Design review of the part built by this model. Coordinates are the model's own, in mm. A direction names the side the tool comes from. Coordinates: 2 decimals unless noted, no trailing zeros. Write each loop counter-clockwise with the first axis right and the second up, starting at its lowest first coordinate (ties: lowest second). Pieces come first, ordered by that corner, then holes. Notation, with made-up numbers: (79.5, 86) - (86.5, 86) arc R22 cw to (86.5, 125) - close; hole circle Ø9 at (-31.75, 19). An arc over 180 degrees is marked (long way). Answer as a JSON object with one key per item and string values.
Autodesk Inventor part; units mm, degrees
ref_plane "YZ Plane" through (0, 0, 0) normal (1, 0, 0) x (0, 1, 0)
ref_plane "XZ Plane" through (0, 0, 0) normal (0, 1, 0) x (-1, 0, 0)
ref_plane "XY Plane" through (0, 0, 0) normal (0, 0, 1) x (1, 0, 0)
sketch "Boceto1" plane through (0, 0, 0) normal (0, 1, 0) x (-1, 0, 0)
  line L0 (0, 0) -> (250, 0)
  line L1 (250, 0) -> (250, -600)
  line L2 (250, -600) -> (0, -600)
  line L3 (0, -600) -> (0, 0)
  line L4 (250, 0) -> (250, -20)
  line L5 (250, -20) -> (0, -20)
  line L6 (0, 0) -> (20, 0)
  line L7 (20, 0) -> (20, -600)
  line L8 (0, -600) -> (0, -580)
  line L9 (0, -580) -> (250, -580)
  line L10 (250, -600) -> (230, -600)
  line L11 (230, -600) -> (230, 0)
  point P0 (20, -20)
  point P1 (20, -580)
  point P2 (230, -580)
  point P3 (230, -20)
  dimension "d0" = 250
  dimension "d1" = 600
  dimension "d2" = 20
  dimension "d3" = 20
  dimension "d4" = 20
  dimension "d5" = 20
extrude "Extrusión1" add sketch "Boceto1" along normal blind 1160 contours L0 L7 L5 L3 | L0 L1 L5 L11 | L9 L7 L2 L3 | L9 L1 L2 L11
extrude "Extrusión2" add sketch "Boceto1" along normal blind 1160 contours L0 L11 L5 L7 | L5 L7 L9 L3 | L5 L11 L9 L7 | L5 L1 L9 L11 | L9 L11 L2 L7
extrude "Extrusión3" cut sketch "Boceto1" along normal blind 1147.5 contours L0 L11 L5 L7 | L5 L7 L9 L3 | L5 L11 L9 L7 | L5 L1 L9 L11 | L9 L11 L2 L7
extrude "Extrusión4" add sketch "Boceto1" along normal blind 787.5 contours L0 L11 L5 L7 | L5 L7 L9 L3 | L5 L11 L9 L7 | L5 L1 L9 L11 | L9 L11 L2 L7
extrude "Extrusión5" cut sketch "Boceto1" along normal blind 775 contours L0 L11 L5 L7 | L5 L7 L9 L3 | L5 L11 L9 L7 | L5 L1 L9 L11 | L9 L11 L2 L7
extrude "Extrusión6" add sketch "Boceto1" along normal blind 470 contours L0 L11 L5 L7 | L5 L7 L9 L3 | L5 L11 L9 L7 | L5 L1 L9 L11 | L9 L11 L2 L7
extrude "Extrusión7" cut sketch "Boceto1" along normal blind 457.5 contours L0 L11 L5 L7 | L5 L7 L9 L3 | L5 L11 L9 L7 | L5 L1 L9 L11 | L9 L11 L2 L7
extrude "Extrusión8" add sketch "Boceto1" along normal blind 152.5 contours L0 L11 L5 L7 | L5 L7 L9 L3 | L5 L11 L9 L7 | L5 L1 L9 L11 | L9 L11 L2 L7
extrude "Extrusión9" cut sketch "Boceto1" along normal blind 140 contours L0 L11 L5 L7 | L5 L7 L9 L3 | L5 L11 L9 L7 | L5 L1 L9 L11 | L9 L11 L2 L7
(1) For pin 1 (1.5 mm diameter, centred on x = -104.5, z = -253, fed in from -Y), flat-tipped, find the tip position at first contact; note if it passes through.
Solved:
{"pin 1": "stops at y = 140"}
(2) Take a section at B-B, the plane y = 405. Write out the cut boundary in (x, z).
Solved:
{"outline": "(-250, -600) - (-230, -600) - (-230, -580) - (-250, -580) - close; (-250, -20) - (-230, -20) - (-230, 0) - (-250, 0) - close; (-20, -600) - (0, -600) - (0, -580) - (-20, -580) - close; (-20, -20) - (0, -20) - (0, 0) - (-20, 0) - close"}
(3) To check wall thickness, follow line 1 (Y direction, x = -200, z = -174.5). State the ranges of the line that lie inside material, in increasing order. Write a range as from..to.
Solved:
{"line 1": "y = 140..152.5, 457.5..470, 775..787.5, 1147.5..1160"}
(4) Take a section at A-A, the plane x = -38. Write out the cut boundary in (y, z).
Solved:
{"outline": "(140, -600) - (152.5, -600) - (152.5, 0) - (140, 0) - close; (457.5, -600) - (470, -600) - (470, 0) - (457.5, 0) - close; (775, -600) - (787.5, -600) - (787.5, 0) - (775, 0) - close; (1147.5, -600) - (1160, -600) - (1160, 0) - (1147.5, 0) - close"}
(5) The part is to be moulded in two halves that separate along Z. For faces 5 (the face through (-240, 0, -10)), 6 (the face through (-10, 303, -580)), say which applies: pulls with the +Z half, pulls with the -Z half, needs draft (parallel to the pull), parting line crosses it, or undercut.
Solved:
{"face 5": "needs draft", "face 6": "undercut"}
(6) Tool access review of faces 1 (the face through (-230, 620, -10)), 2 (the face through (-10, 69, -20)), 3 (the face through (-230, 69, -590)), 4 (the face through (-10, 620, -20)): name each direction out of +Z, -Z, +X, -X, +Y, -Y from which nothing blocks a thin tool from reaching the whole face with its end or side.
Solved:
{"face 1": "+Z, -Z", "face 2": "+X, -X, -Y", "face 3": "+Z, -Z, -Y", "face 4": "+X, -X"}
